Here's how the part is built. I have some questions about the finished solid (model axes, mm). A direction names the side the tool comes from. Round coordinates to 2 decimals unless told otherwise and drop trailing zeros. Order: outer loops, then holes, each group sorted by start corner. A loop starts at its lowest first (then second) coordinate and runs counter-clockwise, first axis right, second up. Notation, with made-up numbers: (50.25, -7) -> (70.25, -7) arc R16 cw to (70.25, 20) -> close; hole circle Ø1 at (13.5, 68.25). An arc over 180 degrees is marked (long way). Use a Markdown table: item, result. Add a question column.
(1) If I drill on probe 1 along Z at (x, y) = (-43.5, 0.5); probe 2 along Y at (x, z) = (190.5, 12.15), over which ranges is the centre line in solid material (lowest first)?
(2) On a 3-axis mill with a long thin cutter (end or side, diameter ignored), from which of +Z, -Z, +X, -X, +Y, -Y can I reach the whole of each face in a straight line? I mean faces 5 (the face through (-3, 12.7, 0)), 6 (the face through (-3, 0, 11.112)). Say none if no direction works.
(3) I want a section at A-A, the plane y = -7. Please give me the cut outline in (x, z), then the cut area to 3 significant figures.
(4) I want a section at C-C, the plane x = 41.5. Please give me the cut outline in (y, z), then the cut area to 3 significant figures.
(5) Thinking about a two-plate mould opening in Z: for faces 1 (the face through (-3, 11.112, 0)), 2 (the face through (-3, -12.7, 0)), 3 (the face through (-3, 0, 12.7)), 4 (the face through (-3, -11.112, 0)), which applies, pulls with the +Z half, pulls with the -Z half, needs draft (parallel to the pull), parting line crosses it, or undercut?
from build123d import *

# Parameters (mm, degrees)
BOSS_EXTRUDE1_DEPTH        = 203.2
BOSS_EXTRUDE1_DEPTH_BACK   = 203.2
SKETCH1_W                  = 25.4
SKETCH1_H                  = 25.4
SKETCH1_W_2                = 22.225
SKETCH1_H_2                = 22.225
F_7_0_201_DIAMETER_HOLE2_D = 5.1054


with BuildPart() as part:
    # Sketch1 → Boss-Extrude1 (new, two sides: drawn at the far end of the back side and taken through both)
    with BuildSketch(Plane(origin=(0, 0, 0), x_dir=(0, 0, -1), z_dir=(1, 0, 0)).offset(-BOSS_EXTRUDE1_DEPTH_BACK)):
        Rectangle(SKETCH1_W, SKETCH1_H)
        Rectangle(SKETCH1_W_2, SKETCH1_H_2, mode=Mode.SUBTRACT)
    extrude(amount=BOSS_EXTRUDE1_DEPTH + BOSS_EXTRUDE1_DEPTH_BACK)

    # #7 (0.201) Diameter Hole2 (through all)
    with Locations(Plane.XY.offset(12.7)):
        with Locations((190.5, 0), (165.1, 0), (139.7, 0), (-139.7, 0), (-165.1, 0), (-190.5, 0)):
            Hole(F_7_0_201_DIAMETER_HOLE2_D / 2)


solid = part.part
Taken from the geometry:
| question | item | result |
|---|---|---|
| 1 | probe 1 | z = -12.7 to -11.11, 11.11 to 12.7 |
| 1 | probe 2 | y = -12.7 to -2.55, 2.55 to 12.7 |
| 2 | face 5 | +Z, -Z, +X, -X, +Y |
| 2 | face 6 | +X, -X |
| 3 | outline | (-203.2, -12.7) -> (203.2, -12.7) -> (203.2, -11.11) -> (-203.2, -11.11) -> close; (-203.2, 11.11) -> (203.2, 11.11) -> (203.2, 12.7) -> (-203.2, 12.7) -> close |
| 3 | area | 1,290 mm2 |
| 4 | outline | (-12.7, -12.7) -> (12.7, -12.7) -> (12.7, 12.7) -> (-12.7, 12.7) -> close; hole (-11.11, -11.11) -> (11.11, -11.11) -> (11.11, 11.11) -> (-11.11, 11.11) -> close |
| 4 | area | 151 mm2 |
| 5 | face 1 | undercut |
| 5 | face 2 | needs draft |
| 5 | face 3 | pulls with the +Z half |
| 5 | face 4 | undercut |
